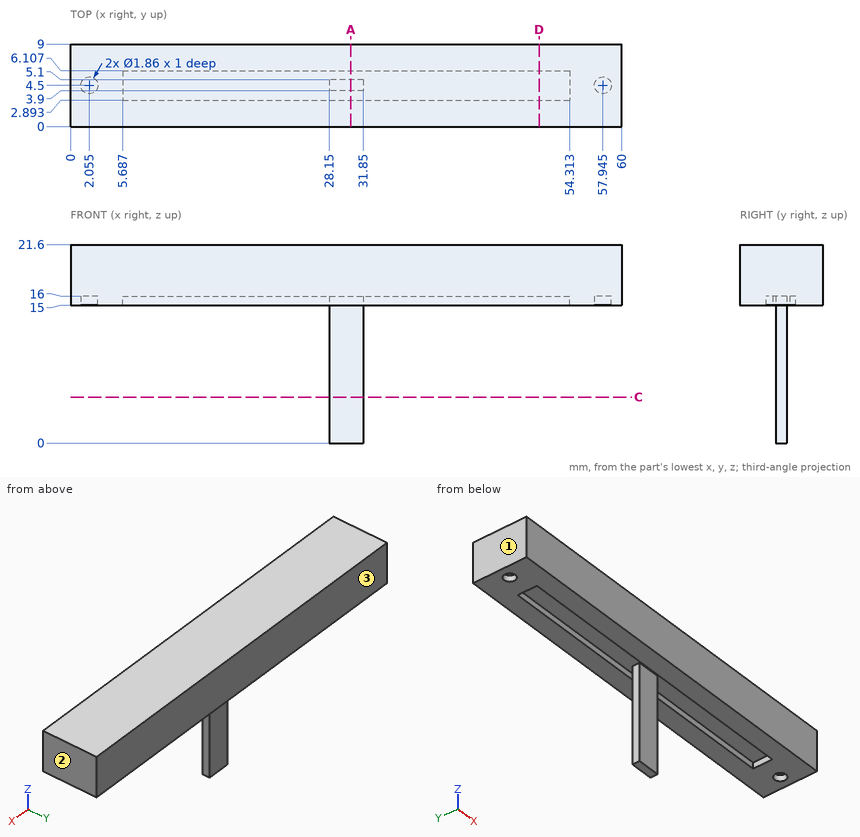
Geometry check sheet. Reference: drawing and pictorial views, mm from the part's lowest x, y, z. Coordinates: 2 decimals unless noted, no trailing zeros. Write each loop counter-clockwise with the first axis right and the second up, starting at its lowest first coordinate (ties: lowest second). Pieces come first, ordered by that corner, then holes. Notation, with made-up numbers: (58, 26.5) -> (72, 26.5) arc R10 ccw to (72, 38.5) -> close; hole circle Ø4 at (62.5, 50.5). An arc over 180 degrees is marked (long way). One line per question, with ' | ' between items.
1. Cross-section at C-C on z = 5. Record the cut outline in (x, y).
Answers:
outline: (28.15, 3.9) -> (31.85, 3.9) -> (31.85, 5.1) -> (28.15, 5.1) -> close
2. Cross-section at D-D on x = 51. Record the cut outline in (y, z), and give its area (3 significant figures).
Answers:
outline: (0, 15) -> (2.89, 15) -> (2.89, 16) -> (6.11, 16) -> (6.11, 15) -> (9, 15) -> (9, 21.6) -> (0, 21.6) -> close | area: 56.2 mm²
3. Depth check by flat-ended pin: pin 1 Ø3 at (x, y) = (7.5, 2.5) entering from -Z; pin 2 Ø1.9 at (x, z) = (30.5, 6.5) entering from +Y; pin 3 Ø1 at (x, y) = (40.5, 4.5) entering from -Z; pin 4 Ø3 at (x, z) = (11, 13) entering from +Y. Enter the tip coordinate at first touch or a pass-through.
Answers:
pin 1: stops at z = 15 | pin 2: stops at y = 5.1 | pin 3: stops at z = 16 | pin 4: passes through
4. Cross-section at A-A on x = 30.5. Record the cut outline in (y, z).
Answers:
outline: (0, 15) -> (2.89, 15) -> (2.89, 16) -> (3.9, 16) -> (3.9, 0) -> (5.1, 0) -> (5.1, 16) -> (6.11, 16) -> (6.11, 15) -> (9, 15) -> (9, 21.6) -> (0, 21.6) -> close
5. Draft check along X on the marked faces 1, 2 and 3. Enter one of: +X half, -X half, draft (parallel to the pull), parting line (faces both ways), or undercut.
Answers:
face 1: -X half | face 2: +X half | face 3: draft
6. Thickness scan on probe 1 along X at (y, z) = (4.75, 7); probe 2 along Z at (x, y) = (7, 7.75); probe 3 along Z at (x, y) = (46.5, 4.5). Record the ranges inside material, lowest first. Write a range as from..to.
Answers:
probe 1: x = 28.15..31.85 | probe 2: z = 15..21.6 | probe 3: z = 16..21.6
